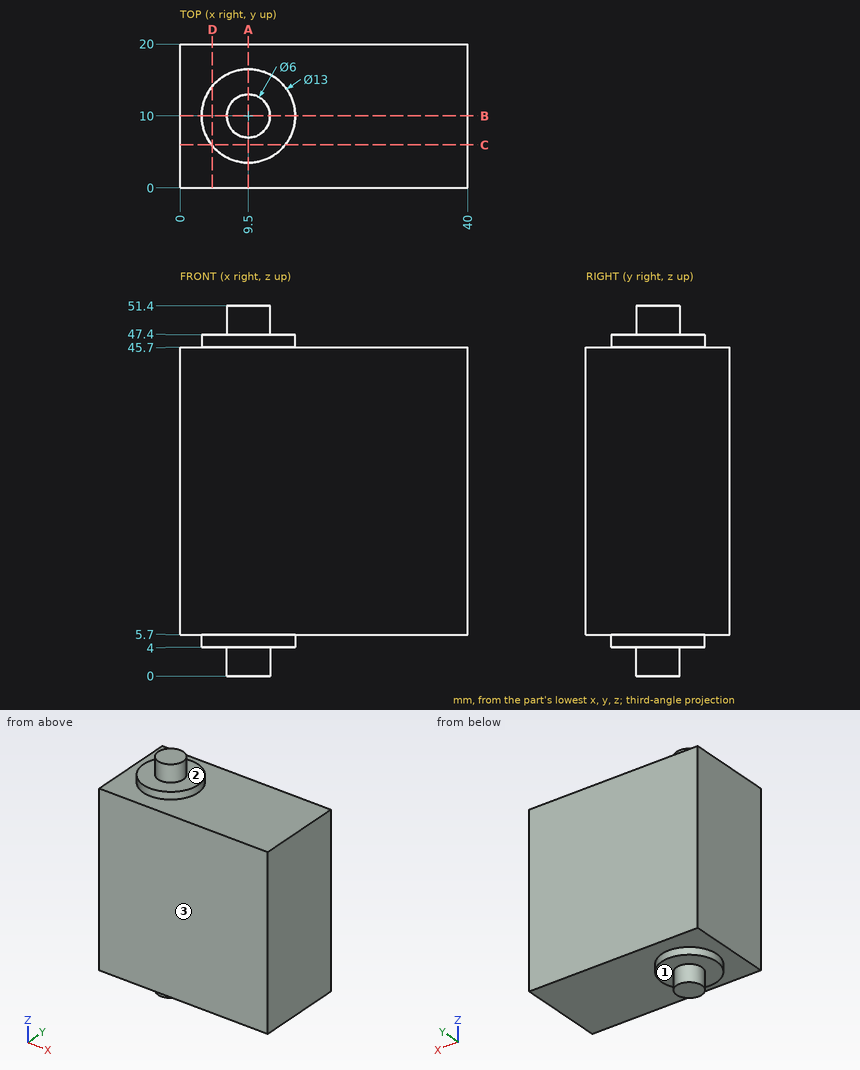
Here's the drawing with two shaded views (mm, measured from the low corner). I have some questions. A direction names the side the tool comes from. Give positions to 0.01 mm unless a question says otherwise; leave off trailing zeros. Order: outer loops, then holes, each group sorted by start corner. A loop starts at its lowest first (then second) coordinate and runs counter-clockwise, first axis right, second up. Notation, with made-up numbers: (-16, 27) -> (5, 27) arc R11 cw to (5, 32) -> close; hole circle Ø3 at (59.25, -10). An arc over 180 degrees is marked (long way). Use a Markdown table: item, result. Add a question column.
Item 1: For the marked faces 1, 2 and 3, which set-ups out of +Z, -Z, +X, -X, +Y, -Y let a thin tool reach every point of the face, with its end or its side?
Item 2: Imagine slicing it at C-C on y = 6. Please give me the cut outline in (x, z).
Item 3: Imagine slicing it at B-B on y = 10. Please give me the cut outline in (x, z).
Item 4: Imagine slicing it at D-D on x = 4.5. Please give me the cut outline in (y, z).
Item 5: Will these pins go through, and if not, where does the flat tip stop? pin 1 (12 mm diameter, centred on x = 27, y = 15, fed in from -Z); pin 2 (4 mm diameter, centred on x = 27, y = 6, fed in from +Z).
Item 6: Imagine slicing it at A-A on x = 9.5. Please give me the cut outline in (y, z), plus the area to 3 significant figures.
Item 7: I need wall thicknesses on line 1 (Z direction, x = 2.5, y = 7); line 2 (Z direction, x = 13, y = 10.5). Which ranges of each line are inside material? Lowest first, please.
Data:
| question | item | result |
|---|---|---|
| 1 | face 1 | -Z |
| 1 | face 2 | +Z |
| 1 | face 3 | +Z, -Z, +X, -X, -Y |
| 2 | outline | (0, 5.7) -> (4.38, 5.7) -> (4.38, 4) -> (14.62, 4) -> (14.62, 5.7) -> (40, 5.7) -> (40, 45.7) -> (14.62, 45.7) -> (14.62, 47.4) -> (4.38, 47.4) -> (4.38, 45.7) -> (0, 45.7) -> close |
| 3 | outline | (0, 5.7) -> (3, 5.7) -> (3, 4) -> (6.5, 4) -> (6.5, 0) -> (12.5, 0) -> (12.5, 4) -> (16, 4) -> (16, 5.7) -> (40, 5.7) -> (40, 45.7) -> (16, 45.7) -> (16, 47.4) -> (12.5, 47.4) -> (12.5, 51.4) -> (6.5, 51.4) -> (6.5, 47.4) -> (3, 47.4) -> (3, 45.7) -> (0, 45.7) -> close |
| 4 | outline | (0, 5.7) -> (5.85, 5.7) -> (5.85, 4) -> (14.15, 4) -> (14.15, 5.7) -> (20, 5.7) -> (20, 45.7) -> (14.15, 45.7) -> (14.15, 47.4) -> (5.85, 47.4) -> (5.85, 45.7) -> (0, 45.7) -> close |
| 5 | pin 1 | stops at z = 5.7 |
| 5 | pin 2 | stops at z = 45.7 |
| 6 | outline | (0, 5.7) -> (3.5, 5.7) -> (3.5, 4) -> (7, 4) -> (7, 0) -> (13, 0) -> (13, 4) -> (16.5, 4) -> (16.5, 5.7) -> (20, 5.7) -> (20, 45.7) -> (16.5, 45.7) -> (16.5, 47.4) -> (13, 47.4) -> (13, 51.4) -> (7, 51.4) -> (7, 47.4) -> (3.5, 47.4) -> (3.5, 45.7) -> (0, 45.7) -> close |
| 6 | area | 892 mm² |
| 7 | line 1 | z = 5.7 to 45.7 |
| 7 | line 2 | z = 4 to 47.4 |
